```python
from build123d import *

# Parameters (mm, degrees)
BOSS_EXTRUDE1_DEPTH     = 30
BOSS_EXTRUDE1_TAPER     = -26.56505118
SKETCH3_OUTSIDE_W       = 108.076
SKETCH3_OUTSIDE_H       = 105.2
CUT_EXTRUDE1_DEPTH      = 30
CUT_EXTRUDE1_TAPER      = 26.56505118
SKETCH5_R               = 19.347524159
CUT_EXTRUDE2_DEPTH      = 25
SHELL1_T                = -2
SKETCH6_R               = 4
SKETCH6_R_2             = 2
BOSS_EXTRUDE2_DEPTH     = 13
SKETCH10_R              = 6
SKETCH10_R_2            = 4
BOSS_EXTRUDE4_DEPTH     = 3
FILLET5_R               = 1.5
CUT_EXTRUDE3_START      = -1
CUT_EXTRUDE3_DEPTH      = 2
CUT_EXTRUDE3_DEPTH_BACK = 2
FILLET6_R               = 1.5


with BuildPart() as part:
    # Sketch1 → Boss-Extrude1 (new body)
    with BuildSketch(Plane(origin=(0, 0, 0), x_dir=(1, 0, 0), z_dir=(0, 1, 0))):
        Polygon((0, 12.360679775), (-11.755705046, 3.819660113), (-7.26542528, -10), (7.26542528, -10), (11.755705046, 3.819660113), align=None)
    extrude(amount=BOSS_EXTRUDE1_DEPTH, taper=BOSS_EXTRUDE1_TAPER)

    # Sketch3 outside → Cut-Extrude1 (cut)
    with BuildSketch(Plane(origin=(0, 30, 0), x_dir=(1, 0, 0), z_dir=(0, 1, 0))):
        with Locations((0, 2.951)):
            Rectangle(SKETCH3_OUTSIDE_W, SKETCH3_OUTSIDE_H)
        Polygon((7.26542528, 10), (-7.26542528, 10), (-11.755705046, -3.819660113), (0, -12.360679775), (11.755705046, -3.819660113), align=None, mode=Mode.SUBTRACT)
    extrude(amount=-CUT_EXTRUDE1_DEPTH, taper=CUT_EXTRUDE1_TAPER, mode=Mode.SUBTRACT)

    # Sketch5 → Cut-Extrude2 (cut)
    with BuildSketch(Plane(origin=(0, 15, 0), x_dir=(1, 0, 0), z_dir=(0, 1, 0))):
        Circle(SKETCH5_R)
    extrude(amount=CUT_EXTRUDE2_DEPTH, mode=Mode.SUBTRACT)

    # Shell1
    shell1_openings = [part.faces().sort_by_distance(p)[0] for p in [
        (0, 15, 0),
    ]]
    offset(amount=SHELL1_T, openings=shell1_openings, kind=Kind.INTERSECTION)

    # Sketch6 → Boss-Extrude2 (add)
    with BuildSketch(Plane(origin=(0, 2, 0), x_dir=(1, 0, 0), z_dir=(0, 1, 0))):
        Circle(SKETCH6_R)
        Circle(SKETCH6_R_2, mode=Mode.SUBTRACT)
    extrude(amount=BOSS_EXTRUDE2_DEPTH)

    # Sketch12 → Loft1 section 0
    with BuildSketch(Plane(origin=(0, 3, 0), x_dir=(1, 0, 0), z_dir=(0, 1, 0))):
        Polygon((0, 11.450849719), (-10.890405242, 3.538507163), (-6.730640591, -9.263932023), (6.730640591, -9.263932023), (10.890405242, 3.538507163), align=None)
    # Sketch13 → Loft1 section 1
    with BuildSketch(Plane(origin=(0, 2, 0), x_dir=(1, 0, 0), z_dir=(0, 1, 0))):
        Polygon((10.30261999, 3.347524158), (0, 10.83281573), (-10.30261999, 3.347524158), (-6.367369327, -8.763932023), (6.367369327, -8.763932023), align=None)
    loft()

    # Sketch10 → Boss-Extrude4 (add)
    with BuildSketch(Plane(origin=(0, 3, 0), x_dir=(1, 0, 0), z_dir=(0, 1, 0))):
        Circle(SKETCH10_R)
        Circle(SKETCH10_R_2, mode=Mode.SUBTRACT)
    extrude(amount=BOSS_EXTRUDE4_DEPTH)

    # Fillet5
    fillet5_edges = [part.edges().sort_by_distance(p)[0] for p in [
        (-6, 3, 0),
        (-4, 6, 0),
    ]]
    fillet(fillet5_edges, radius=FILLET5_R)

    # Sketch10<3> → Cut-Extrude3 (cut, two sides)
    with BuildSketch(Plane(origin=(0, 3, 0), x_dir=(1, 0, 0), z_dir=(0, 1, 0)).offset(CUT_EXTRUDE3_START)) as cut_extrude3_sk:
        Polygon((0, 5.196152423), (-4.5, 2.598076211), (-4.5, -2.598076211), (0, -5.196152423), (4.5, -2.598076211), (4.5, 2.598076211), align=None)
    extrude(amount=CUT_EXTRUDE3_DEPTH, mode=Mode.SUBTRACT)
    extrude(cut_extrude3_sk.sketch, amount=-CUT_EXTRUDE3_DEPTH_BACK, mode=Mode.SUBTRACT)

    # Fillet6
    fillet6_edges = [part.edges().sort_by_distance(p)[0] for p in [
        (-6, 6, 0),
        (4.5, 4, 0),
        (2.25, 4, 3.897114317),
        (-2.25, 4, 3.897114317),
        (-4.5, 4, 0),
        (-2.25, 4, -3.897114317),
        (2.25, 4, -3.897114317),
    ]]
    fillet(fillet6_edges, radius=FILLET6_R)


solid = part.part
```
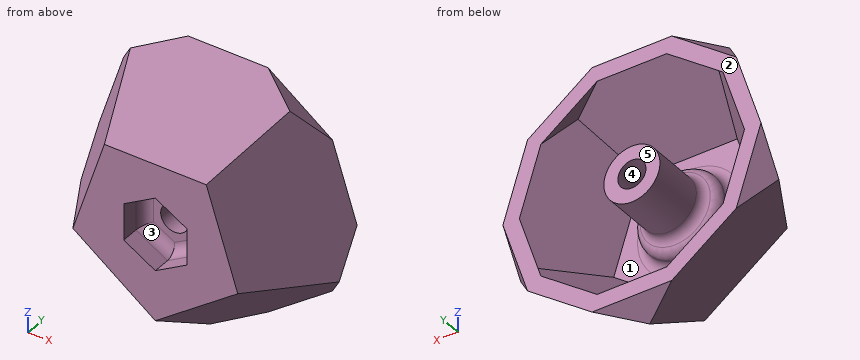
The listing builds one solid part. Answer for the finished solid, in the listing's coordinates (mm). Face numbers are marked on the shaded views. A direction names the side the tool comes from. Coordinates: 2 decimals unless noted, no trailing zeros. One line per item, written item: value.
1) Each of these flat-tipped pins is pushed along its axis until it touches: pin 1 Ø5 at (x, z) = (-1.5, 1) entering from -Y; pin 2 Ø2 at (y, z) = (9, -0.5) entering from -X; pin 3 Ø2 at (x, z) = (-10, 6.5) entering from +Y; pin 4 Ø2.5 at (x, z) = (0, 0) entering from +Y. Where does it stop, or does it pass through?
Geometry check:
pin 1: stops at y = 3.5
pin 2: stops at x = -16.03
pin 3: stops at y = 9.51
pin 4: passes through
2) Find section A-A (y = 10.25). Count the separate pieces of the cut face and the enclosed holes in it, and give its area (3 significant figures).
Geometry check:
separate pieces: 2
enclosed holes: 2
area: 265 mm2
3) For a pull along X with two mould halves and no side action, classify the marked faces 4 and 5 as pulls with the +X half, pulls with the -X half, needs draft (parallel to the pull), parting line crosses it, or undercut.
Geometry check:
face 4: undercut
face 5: needs draft
4) Consider line 1 along X through (y, z) = (11.5, 0); line 2 along X through (y, z) = (8.5, 0); line 3 along Z through (x, y) = (0, 12.5). Determine where each line is inside the solid, lowest interval first. Write a range as from..to.
Geometry check:
line 1: x = -16.56..-14.21, -4..-2, 2..4, 14.21..16.56
line 2: x = -14.98..-12.63, -4..-2, 2..4, 12.63..14.98
line 3: z = -18.75..-16.51, -4..-2, 2..4, 14.01..16.25
5) A tool of negligible diameter and unlimited length cuts with its end or side. For the marked faces 1, 2 and 3, from which of +Z, -Z, +X, -X, +Y, -Y can it reach the whole face along a straight path? Write none if from no direction.
Geometry check:
face 1: +Y
face 2: +Z, -Z, +X, -X, +Y
face 3: -Y
